Could you check a few things on this model? Use its own coordinates, in mm. A direction names the side the tool comes from. Round coordinates to 2 decimals unless told otherwise and drop trailing zeros. Loops run counter-clockwise (first coordinate to the right, second up) from the corner with the lowest first, then second, coordinate; pieces in that order, holes last. Notation, with made-up numbers: (42, 9) -> (75, 9) arc R16 ccw to (75, 27) -> close; hole circle Ø9 at (54, 1). An arc over 180 degrees is marked (long way). Put each result on its own line as item: value. Start each with the question number.
1. I need wall thicknesses on line 1 (X direction, y = 0, z = 1.15); line 2 (X direction, y = 0, z = 2.75); line 3 (Y direction, x = 20, z = 0.75). Which ranges of each line are inside material? Lowest first, please. Write a range as [from, to].
2. I'm going to push flat-ended pins straight in: P1, Ø1, axis at x = -37.5, z = 1.5, coming from the -Y side; P2, Ø2, axis at y = -47, z = 0.5, coming from the +X side. Where does each tip first touch, or does it pass through?
3. Which directions (+Z, -Z, +X, -X, +Y, -Y) give clear straight access to the entire face, cutting with the end or side of a thin tool? Please do faces 4 (the flat face through (39, -39, 4.572)), 5 (the flat face through (0.055, 58, 2)).
4. If we mould it in two halves opening along X, with no side actions, what happens to faces 1 (the flat face through (-37, 41, 0)), 2 (the conical face through (-2.89, -58.99, 4.45)), 3 (the flat face through (0.563, 58, 2))? For each: pulls with the +X half, pulls with the -X half, needs draft (parallel to the pull), parting line crosses it, or undercut.
5. Imagine slicing it at A-A, the plane y = 0. Please give me the cut outline in (x, z), and give its area (3 significant figures).
6. Imagine slicing it at B-B, the plane z = 0.75. Please give me the cut outline in (x, y), and give its area (3 significant figures).
```python
from build123d import *

# Parameters (mm, degrees)
F1_DEPTH = 4.572
F2_SIZE  = 2.54


with BuildPart() as f1:
    # F0 (on Top) → F1 (new body)
    with BuildSketch(Plane.XY):
        with BuildLine():
            ThreePointArc((0.56272, 54.861114), (-0.308723, -54.863131), (0.05472, 54.863973))
            Line((0.05472, 54.863973), (0.05472, 61.477178))
            ThreePointArc((0.05472, 61.477178), (-0.308722, -61.476427), (0.56272, 61.474627))
            Line((0.56272, 61.474627), (0.56272, 54.861114))
        make_face()
    extrude(amount=F1_DEPTH)

    # F2
    f2_edges = [f1.edges().sort_by_distance(p)[0] for p in [
        (-0.308722, -61.476427, 4.572),
    ]]
    chamfer(f2_edges, length=F2_SIZE)


solid = f1.part
```
Entries:
1. line 1: [-61.48, -54.86], [54.86, 61.48]
1. line 2: [-60.76, -54.86], [54.86, 60.76]
1. line 3: [-58.13, -51.09], [51.09, 58.13]
2. P1: y = -49.1
2. P2: x = 40.79
3. face 4: +Z, +X, -X, +Y, -Y
3. face 5: +Z, -Z, +Y
4. face 1: needs draft
4. face 2: parting line crosses it
4. face 3: undercut
5. outline: (-61.48, 0) -> (-54.86, 0) -> (-54.86, 4.57) -> (-58.94, 4.57) -> (-61.48, 2.03) -> close; (54.86, 0) -> (61.48, 0) -> (61.48, 2.03) -> (58.94, 4.57) -> (54.86, 4.57) -> close
5. area: 54.0 mm^2
6. outline: (0.05, 54.86) -> (0.05, 61.48) arc R61.48 ccw (long way) to (0.56, 61.47) -> (0.56, 54.86) arc R54.86 cw (long way) to start
6. area: 2,410 mm^2
